Geometry check sheet. Reference: the model listing, model coordinates, mm. A direction names the side the tool comes from. Round coordinates to 2 decimals unless told otherwise and drop trailing zeros. Order: outer loops, then holes, each group sorted by start corner. A loop starts at its lowest first (then second) coordinate and runs counter-clockwise, first axis right, second up.
(1) Set-up check for faces 4 (the face through (255.444, 17.764, 5.594)), 5 (the face through (310.391, -31, -21)), 6 (the face through (317.786, -5.402, -41.146)): record each of +Z, -Z, +X, -X, +Y, -Y from which the full face is reachable in a straight line by a thin tool's end or side.
(2) Cross-section at A-A on y = 0. Enter the section's corners in (x, z) (1 decimal).
(3) Gauge pin test, flat ends, axial feed: P1, Ø5, axis at x = 267, y = 3, coming from the +Z side; P2, Ø4, axis at x = 259, z = 4, coming from the +Y side; P3, Ø12, axis at x = 208, y = 18.5, coming from the -Z side. Record the tip position at first contact, or that the pin passes through.
(4) Draft check along X on faces 1 (the face through (190.03, -11.79, -53.08)), 2 (the face through (256.74, -18.75, -14.37)), 3 (the face through (236.29, -6.24, 28.12)). Enter one of: pulls with the +X half, pulls with the -X half, needs draft (parallel to the pull), parting line crosses it, or undercut.
(5) Cross-section at C-C on x = 274.5. Enter the section's corners in (y, z), and give its area (3 significant figures).
(6) Cross-section at D-D on x = 289. Enter the section's corners in (y, z), and give its area (3 significant figures).
(7) Thickness scan on L1, parallel to Z at x = 255.2, y = 0; L2, parallel to Z at x = 190, y = 0 (3 decimals); L3, parallel to Y at x = 203, z = -8. Record the ranges inside material, lowest first.
Autodesk Inventor part; units mm, degrees
ref_plane "YZ Plane" through (0, 0, 0) normal (1, 0, 0) x (0, 1, 0)
ref_plane "XZ Plane" through (0, 0, 0) normal (0, 1, 0) x (-1, 0, 0)
ref_plane "XY Plane" through (0, 0, 0) normal (0, 0, 1) x (1, 0, 0)
sketch "Sketch1" plane through (0, 0, 0) normal (0, 0, 1) x (1, 0, 0)
  line L0 (0, 0) -> (0, 54.375)
  line L1 (0, 54.375) -> (20, 54.375)
  line L2 (0, 0) -> (772.3927, 0)
  line L3 (253.9225, 18.624) -> (253.9225, 0) construction
  line L4 (192, 54.375) -> (253.9225, 18.624)
  line L5 (253.9225, 18.624) -> (256.9225, 18.624)
  line L6 (256.9225, 18.624) -> (325.3908, 36.97)
  line L7 (325.3908, 36.97) -> (325.3908, 0)
  line L8 (192, 54.375) -> (192, 0)
  line L9 (0, 54.375) -> (0, 74.375)
  line L10 (0, 74.375) -> (20, 74.375)
  line L11 (20, 74.375) -> (20, 58.375)
  line L12 (20, 58.375) -> (172, 58.375)
  line L13 (192, 54.375) -> (192, 74.375) construction
  line L14 (325.3908, 36.4995) -> (325.3908, 41.4995)
  line L15 (207, 50.3335) -> (253.2623, 23.624)
  line L16 (260.128, 23.624) -> (310.3908, 37.0919)
  line L17 (253.2623, 23.624) -> (260.128, 23.624)
  line L18 (310.3908, 41.4995) -> (310.3908, 37.0919)
  line L19 (207, 45.7147) -> (207, 21.1203)
  line L20 (325.3908, 36.4995) -> (325.3908, 41.4995)
  line L21 (325.3908, 41.4995) -> (310.3908, 41.4995)
  line L22 (207, 50.3335) -> (192, 58.9938)
  line L23 (207, 50.3335) -> (266.427, 50.3335) construction
  line L24 (172, 58.375) -> (185.0718, 58.375)
  line L25 (192, 58.9938) -> (188, 58.9938)
  line L26 (188, 58.9938) -> (188, 54.375)
  line L27 (188, 54.375) -> (192, 54.375)
  point P0 (255.4225, 18.624)
  dimension "d0" = 54.375
  dimension "d2" = 18.624
  dimension "d3" = 150
  dimension "d4" = 3
  dimension "d5" = 15
  dimension "d6" = 36.97
  dimension "d7" = 518.4701
  dimension "d8" = 20
  dimension "d9" = 20
  dimension "d10" = 16
  dimension "d18" = 4
  dimension "d21" = 5
  dimension "d22" = 15
  dimension "d23" = 150
  dimension "d24" = 4
revolve "Revolution1" add sketch "Sketch1" angle 360 about axis through (0, 0, 0) along (1, 0, 0) contours L27 L26 L25 L22 L15 L17 L16 L18 L21 L14 L6 L5 L4
properties part number "nozzle" material "Stainless Steel, Austenitic"
Found:
1. face 4: +X, -X
1. face 5: none
1. face 6: +X
2. outline: (188, -59) - (192, -59) - (207, -50.3) - (253.3, -23.6) - (260.1, -23.6) - (310.4, -37.1) - (310.4, -41.5) - (325.4, -41.5) - (325.4, -37) - (256.9, -18.6) - (253.9, -18.6) - (192, -54.4) - (188, -54.4) - close; (188, 54.4) - (192, 54.4) - (253.9, 18.6) - (256.9, 18.6) - (325.4, 37) - (325.4, 41.5) - (310.4, 41.5) - (310.4, 37.1) - (260.1, 23.6) - (253.3, 23.6) - (207, 50.3) - (192, 59) - (188, 59) - close
3. P1: stops at z = 26.01
3. P2: stops at y = 23.6
3. P3: stops at z = -50.43
4. face 1: needs draft
4. face 2: undercut
4. face 3: pulls with the -X half
5. outline: circle Ø54.95 at (0, 0); hole circle Ø46.67 at (0, 0)
5. area: 661 mm2
6. outline: circle Ø62.72 at (0, 0); hole circle Ø54.44 at (0, 0)
6. area: 762 mm2
7. L1: z = -23.62 to -18.62, 18.62 to 23.62
7. L2: z = -58.994 to -54.375, 54.375 to 58.994
7. L3: y = -52.03 to -47.35, 47.35 to 52.03
